```python
from build123d import *

# Parameters (mm, degrees)
BOSS_EXTRUDE1_DEPTH = 1000
SKETCH2_W           = 125
SKETCH2_H           = 150
BOSS_EXTRUDE2_DEPTH = 100
SKETCH3_R           = 10
CUT_EXTRUDE1_DEPTH  = 10


with BuildPart() as part:
    # Sketch1 → Boss-Extrude1 (new, symmetric)
    with BuildSketch(Plane.XY):
        Polygon((0, 0), (0, 25), (25, 25), (25, 50), (50, 50), (50, 25), (75, 25), (75, 75), (125, 75), (125, -75), (75, -75), (75, -25), (50, -25), (50, -50), (25, -50), (25, -25), (0, -25), align=None)
    extrude(amount=BOSS_EXTRUDE1_DEPTH, both=True)

    # Sketch2 → Boss-Extrude2 (add)
    with BuildSketch(Plane.XY.offset(1000)):
        with Locations((62.5, 0)):
            Rectangle(SKETCH2_W, SKETCH2_H)
    extrude(amount=BOSS_EXTRUDE2_DEPTH)

    # Sketch3 → Cut-Extrude1 (cut)
    with BuildSketch(Plane(origin=(0, 0, -1000), x_dir=(-1, 0, 0), z_dir=(0, 0, -1))):
        with Locations((-100, 50)):
            Circle(SKETCH3_R)
        with Locations(Location((-100, -50, 0), (0, 0, 180))):
            Circle(SKETCH3_R)
    extrude(amount=-CUT_EXTRUDE1_DEPTH, mode=Mode.SUBTRACT)


solid = part.part
```
Check sheet for the modelled part. Datum: model origin and axes. Units: mm. Give positions to 0.01 mm unless a question says otherwise; leave off trailing zeros. Order: outer loops, then holes, each group sorted by start corner. A loop starts at its lowest first (then second) coordinate and runs counter-clockwise, first axis right, second up. Notation, with made-up numbers: M 35,17.25 L 66,17.25 A4 cw 66,24.25 Z; hole C 35,-13.5 d1. An arc over 180 degrees is marked long. Answer in a Markdown table with one row per item.
1) Cross-section at A-A, the plane z = 301. Enter the section's corners in (x, y), plus the area to 3 significant figures.
Filled sheet:
| item | result |
|---|---|
| outline | M 0,-25 L 25,-25 L 25,-50 L 50,-50 L 50,-25 L 75,-25 L 75,-75 L 125,-75 L 125,75 L 75,75 L 75,25 L 50,25 L 50,50 L 25,50 L 25,25 L 0,25 Z |
| area | 12,500 mm2 |
2) Thickness scan on L1, parallel to Y at x = 100, z = -997; L2, parallel to X at y = -35.5, z = -427; L3, parallel to Z at x = 37, y = 64. Record the ranges inside material, lowest first. Write a range as [from, to].
Filled sheet:
| item | result |
|---|---|
| L1 | y = [-75, -60], [-40, 40], [60, 75] |
| L2 | x = [25, 50], [75, 125] |
| L3 | z = [1000, 1100] |
3) Release check for a two-part mould opening along X. For faces 1 (the flat face through (75, 50, 14)), 2 (the flat face through (103, -75, 35)), 3 (the flat face through (75, -50, 14)), 4 (the flat face through (125, -1, 35)) record: +X half, -X half, draft (parallel to the pull), parting line (faces both ways), or undercut.
Filled sheet:
| item | result |
|---|---|
| face 1 | undercut |
| face 2 | draft |
| face 3 | undercut |
| face 4 | +X half |
4) Gauge pin test, flat ends, axial feed: P1, Ø1, axis at y = 36, z = -388, coming from the -X side; P2, Ø10, axis at x = 104, y = 47.5, coming from the -Z side; P3, Ø5, axis at y = -55.5, z = 679, coming from the -X side. Record the tip position at first contact, or that the pin passes through.
Filled sheet:
| item | result |
|---|---|
| P1 | stops at x = 25 |
| P2 | stops at z = -990 |
| P3 | stops at x = 75 |
